Check sheet for the drawn part. Datum: minimum x, y, z corner. Units: mm. A direction names the side the tool comes from. Give positions to 0.01 mm unless a question says otherwise; leave off trailing zeros. Loops run counter-clockwise (first coordinate to the right, second up) from the corner with the lowest first, then second, coordinate; pieces in that order, holes last.
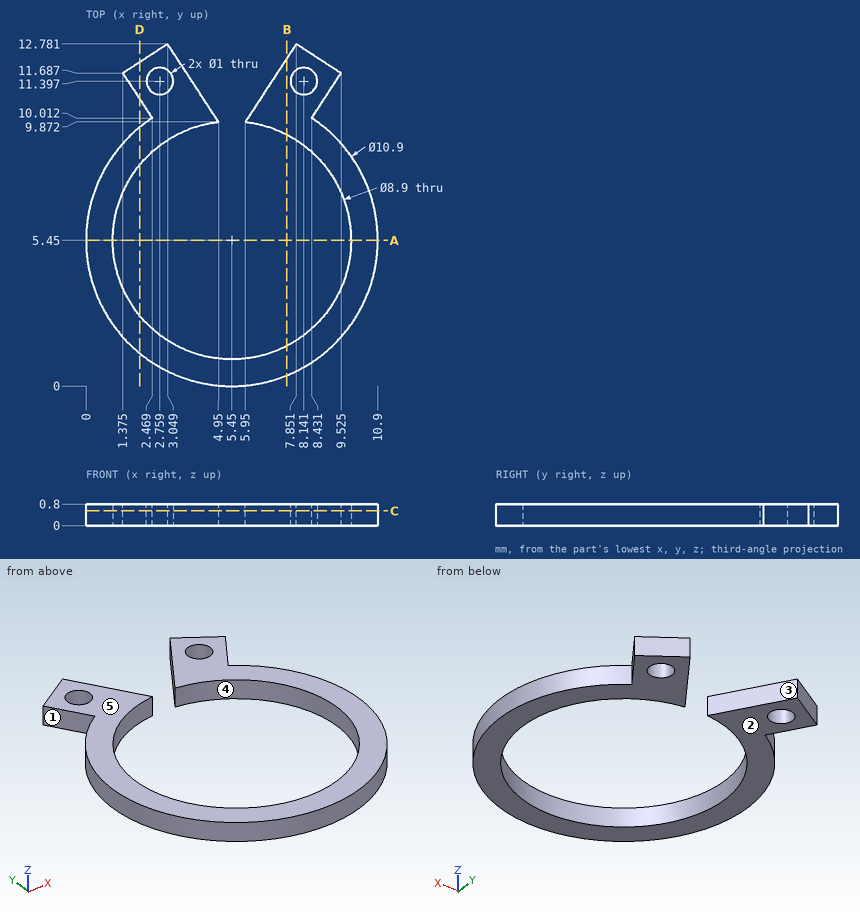
1) Mould release check, pull along Y, two halves, no side actions. Record for the marked faces 3, 4 and 5: +Y half, -Y half, draft (parallel to the pull), parting line (faces both ways), or undercut.
2) Sectioned sample at C-C on z = 0.55. Count the separate pieces of the cut face and the enclosed holes in it.
3) Sectioned sample at B-B on x = 7.5. Enter the section's corners in (y, z) (1 decimal).
4) Sectioned sample at D-D on x = 2. Enter the section's corners in (y, z) (1 decimal).
5) Tool access check on the marked faces 1 and 2. Record the directions out of +Z, -Z, +X, -X, +Y, -Y that give a thin tool (end or side, any length) a straight path to the whole face; none if there is none.
6) Depth check by flat-ended pin: P1, Ø3, axis at x = 4.5, y = 4, coming from the -Z side. Enter the tip coordinate at first touch or a pass-through.
7) Scan lines: line 1 along Y through (x, z) = (1.5, 0.15) (1 decimal); line 2 along X through (y, z) = (5.45, 0.45); line 3 along Y through (x, z) = (9.25, 0.1) (1 decimal). Record each from-to range of solid material in increasing order.
8) Sectioned sample at A-A on y = 5.45. Enter the section's corners in (x, z).
Determined:
1. face 3: +Y half
1. face 4: undercut
1. face 5: draft
2. separate pieces: 1
2. enclosed holes: 2
3. outline: (0.4, 0) - (1.5, 0) - (1.5, 0.8) - (0.4, 0.8) - close; (9.4, 0) - (12.2, 0) - (12.2, 0.8) - (9.4, 0.8) - close
4. outline: (1.2, 0) - (2.6, 0) - (2.6, 0.8) - (1.2, 0.8) - close; (8.3, 0) - (9.7, 0) - (9.7, 0.8) - (8.3, 0.8) - close; (10.7, 0) - (12.1, 0) - (12.1, 0.8) - (10.7, 0.8) - close
5. face 1: +Z, -Z, -X
5. face 2: -Z, +X, -X, +Y, -Y
6. P1: passes through
7. line 1: y = 1.7 to 3.4, 7.5 to 9.2, 11.5 to 11.8
7. line 2: x = 0 to 1, 9.9 to 10.9
7. line 3: y = 1.5 to 3.1, 7.8 to 9.4, 11.3 to 11.9
8. outline: (0, 0) - (1, 0) - (1, 0.8) - (0, 0.8) - close; (9.9, 0) - (10.9, 0) - (10.9, 0.8) - (9.9, 0.8) - close
